from build123d import *

# Parameters (mm, degrees)
BOSS_EXTRUDE1_DEPTH      = 1.25
SKETCH2_W                = 14.25
SKETCH2_H                = 15
BOSS_EXTRUDE2_DEPTH      = 4.6
FILLET1_R                = 3
SKETCH5_W                = 20
SKETCH5_H                = 82.2
BASE_PLATE_DEPTH         = 6
SLOT_CUT_DEPTH           = 82.2
REAR_TAB_DEPTH           = 4.4
REAR_TAB_DEPTH_BACK      = 0.4
SKETCH8_W                = 15.25
SKETCH8_H                = 3
SKETCH22_W               = 15.25
SKETCH22_H               = 3
FRONT_SUPPORT_RAIL_DEPTH = 2.1
SKETCH23_W               = 0.8
SKETCH23_H               = 25
BEND_SLOT_DEPTH          = 91.682082023
SKETCH20_W               = 7.75
SKETCH20_H               = 6
SKETCH20_W_2             = 4.75
BOSS_EXTRUDE3_DEPTH      = 0.45
FILLET6_R                = 2.5
CUT_EXTRUDE4_DEPTH       = 92.879282213
CUT_EXTRUDE5_DEPTH       = 5.2
FILLET5_R                = 1
FILLET7_R                = 0.4
BOSS_EXTRUDE4_DEPTH      = 2
CHAMFER1_SIZE            = 2
FILLET8_R                = 2


# Some blends are built 0.0001 mm under size
with BuildPart() as part:
    # Sketch1 → Boss-Extrude1 (new body)
    with BuildSketch(Plane.XY):
        Polygon((0, 0), (14, 0), (14, 17), (-2, 17), (-2, 0), align=None)
    extrude(amount=BOSS_EXTRUDE1_DEPTH)

    # Sketch2 → Boss-Extrude2 (add)
    with BuildSketch(Plane.XY):
        with Locations((5.125, 7.5)):
            Rectangle(SKETCH2_W, SKETCH2_H)
    extrude(amount=-BOSS_EXTRUDE2_DEPTH)

    # Fillet1
    fillet1_edges = [part.edges().sort_by_distance(p)[0] for p in [
        (12.25, 15, -2.3),
        (14, 17, 0.625),
    ]]
    fillet(fillet1_edges, radius=FILLET1_R)

    # Mirror1: part across plane


with BuildPart() as body_2:
    # Sketch5 → Base Plate (new body)
    with BuildSketch(Plane(origin=(0, 0, 0), x_dir=(1, 0, 0), z_dir=(0, 1, 0))):
        with Locations((10, 45.7)):
            Rectangle(SKETCH5_W, SKETCH5_H)
    extrude(amount=BASE_PLATE_DEPTH)

    # Sketch18 → Slot Cut (cut)
    with BuildSketch(Plane(origin=(0, 0, -86.8), x_dir=(-1, 0, 0), z_dir=(0, 0, -1))):
        Polygon((0, 0.4), (-15.25, 0.4), (-15.25, 2.5), (-17.25, 2.5), (-17.25, 4.5), (-15.25, 6), (0, 6), align=None)
    extrude(amount=-SLOT_CUT_DEPTH, mode=Mode.SUBTRACT)

    # Sketch8 → Rear Tab (add, two sides: drawn at the far end of the back side and taken through both)
    with BuildSketch(Plane(origin=(0, 0.4, 0), x_dir=(1, 0, 0), z_dir=(0, 1, 0)).offset(-REAR_TAB_DEPTH_BACK)):
        with Locations((7.625, 85.3)):
            Rectangle(SKETCH8_W, SKETCH8_H)
    extrude(amount=REAR_TAB_DEPTH + REAR_TAB_DEPTH_BACK)

    # Sketch22 → Front Support Rail (add)
    with BuildSketch(Plane(origin=(0, 0.4, 0), x_dir=(1, 0, 0), z_dir=(0, 1, 0))):
        with Locations((7.625, 6.1)):
            Rectangle(SKETCH22_W, SKETCH22_H)
    extrude(amount=FRONT_SUPPORT_RAIL_DEPTH)

    # Sketch23 → Bend Slot (cut, through all)
    with BuildSketch(Plane(origin=(0, 0, 0), x_dir=(1, 0, 0), z_dir=(0, 1, 0))):
        with Locations((14.85, 74.3)):
            Rectangle(SKETCH23_W, SKETCH23_H)
    extrude(amount=BEND_SLOT_DEPTH, mode=Mode.SUBTRACT)

    # Mirror2: body 2 across plane


with BuildPart() as part_1:
    add(part.part)
    add(part.part.mirror(Plane(origin=(-2, 0, 1.25), x_dir=(0, 0, 1), z_dir=(1, 0, 0))))



with BuildPart() as body_2_1:
    add(body_2.part)
    add(body_2.part.mirror(Plane(origin=(0, 6, -4.6), x_dir=(0, 0, 1), z_dir=(1, 0, 0))))


with BuildPart() as part_2:
    add(part_1.part)

    add(body_2_1.part)  # Boss-Extrude3 merges body 2
    # Sketch20 → Boss-Extrude3 (add)
    with BuildSketch(Plane.XY.offset(-4.6)):
        with Locations((16.125, 3)):
            Rectangle(SKETCH20_W, SKETCH20_H)
        with Locations((-17.625, 3)):
            Rectangle(SKETCH20_W_2, SKETCH20_H)
    extrude(amount=BOSS_EXTRUDE3_DEPTH)

    # Fillet6
    fillet6_edges = [part_2.edges().sort_by_distance(p)[0] for p in [
        (-20, 3, -4.15),
        (20, 3, -4.15),
        (20, 3, -86.8),
        (0, 4.8, -86.8),
        (-20, 3, -86.8),
    ]]
    fillet(fillet6_edges, radius=FILLET6_R)

    # Sketch15 → Cut-Extrude4 (cut, through all)
    with BuildSketch(Plane.XY.offset(1.25)):
        with BuildLine():
            Line((7.5, 5), (-11.5, 5))
            ThreePointArc((-11.5, 5), (-14.5, 8), (-11.5, 11))
            Line((-11.5, 11), (7.5, 11))
            ThreePointArc((7.5, 11), (10.5, 8), (7.5, 5))
        make_face()
    extrude(amount=-CUT_EXTRUDE4_DEPTH, mode=Mode.SUBTRACT)

    # Sketch16 → Cut-Extrude5 (cut)
    with BuildSketch(Plane.XY.offset(1.25)):
        with BuildLine():
            Line((-15.6, 0), (11.6, 0))
            Line((11.6, 0), (11.6, 12))
            ThreePointArc((11.6, 12), (10.911700936, 13.661700936), (9.25, 14.35))
            Line((9.25, 14.35), (-13.25, 14.35))
            ThreePointArc((-13.25, 14.35), (-14.911700936, 13.661700936), (-15.6, 12))
            Line((-15.6, 12), (-15.6, 0))
        make_face()
    extrude(amount=-CUT_EXTRUDE5_DEPTH, mode=Mode.SUBTRACT)

    # Fillet5
    # the kernel refuses this fillet: 1 mm, written as the material it adds along each edge
    with BuildSketch(Plane(origin=(9.25, 14.35, -3.95), x_dir=(0, -1, 0), z_dir=(-1, 0, 0))) as fillet5_piece_1:
        with BuildLine():
            CenterArc((FILLET5_R, FILLET5_R), FILLET5_R, 180, 90)
            Line((0, FILLET5_R), (0, 0))
            Line((0, 0), (FILLET5_R, 0))
        make_face()
    extrude(amount=22.5)
    with BuildSketch(Plane(origin=(-13.25, 12, -3.95), x_dir=(0, 1, 0), z_dir=(1, 0, 0))) as fillet5_piece_2:
        with BuildLine():
            CenterArc((2.35 - FILLET5_R, FILLET5_R), FILLET5_R, 270, 90)
            Line((2.35, FILLET5_R), (2.35, 0))
            Line((2.35, 0), (2.35 - FILLET5_R, 0))
        make_face()
    revolve(axis=Axis((-13.25, 12, -3.95), (0, 0, 1)), revolution_arc=90)
    with BuildSketch(Plane(origin=(-15.6, 12, -3.95), x_dir=(1, 0, 0), z_dir=(0, -1, 0))) as fillet5_piece_3:
        with BuildLine():
            CenterArc((FILLET5_R, FILLET5_R), FILLET5_R, 180, 90)
            Line((0, FILLET5_R), (0, 0))
            Line((0, 0), (FILLET5_R, 0))
        make_face()
    extrude(amount=12)
    with BuildSketch(Plane(origin=(11.6, 0, -3.95), x_dir=(0, 0, 1), z_dir=(0, 1, 0))) as fillet5_piece_4:
        with BuildLine():
            CenterArc((FILLET5_R, -FILLET5_R), FILLET5_R, 90, 90)
            Line((0, -FILLET5_R), (0, 0))
            Line((0, 0), (FILLET5_R, 0))
        make_face()
    extrude(amount=12)
    with BuildSketch(Plane(origin=(9.25, 12, -3.95), x_dir=(1, 0, 0), z_dir=(0, -1, 0))) as fillet5_piece_5:
        with BuildLine():
            CenterArc((2.35 - FILLET5_R, FILLET5_R), FILLET5_R, 270, 90)
            Line((2.35, FILLET5_R), (2.35, 0))
            Line((2.35, 0), (2.35 - FILLET5_R, 0))
        make_face()
    revolve(axis=Axis((9.25, 12, -3.95), (0, 0, 1)), revolution_arc=90)
    with BuildSketch(Plane(origin=(15.25, 0.4, -7.6), x_dir=(0, 0, -1), z_dir=(0, 1, 0))) as fillet5_piece_6:
        with BuildLine():
            CenterArc((FILLET5_R, FILLET5_R), FILLET5_R, 180, 90)
            Line((0, FILLET5_R), (0, 0))
            Line((0, 0), (FILLET5_R, 0))
        make_face()
    extrude(amount=2.1)
    with BuildSketch(Plane(origin=(-15.25, 0.4, -7.6), x_dir=(0, 0, -1), z_dir=(0, 1, 0))) as fillet5_piece_7:
        with BuildLine():
            CenterArc((FILLET5_R, -FILLET5_R), FILLET5_R, 90, 90)
            Line((0, -FILLET5_R), (0, 0))
            Line((0, 0), (FILLET5_R, 0))
        make_face()
    extrude(amount=2.1)
    # the kernel refuses this fillet: 1 mm, written as the material it takes off along each edge
    with BuildSketch(Plane(origin=(17.25, 2.5, -86.8), x_dir=(0.9759656656854916, -1.7336632852602407e-15, 0.21792434330077798), z_dir=(0, 1, 0))) as fillet5_2_piece_1_section:
        with BuildLine():
            CenterArc((1.237684498, -0.954173231), FILLET5_R, 72.587148881, 120)
            Line((0.261718832, -1.172097575), (0.164122266, -1.193890009))
            Line((0.164122266, -1.193890009), (-0.097596567, -0.021792434))
            Line((-0.097596567, -0.021792434), (-0.021792434, 0.097596567))
            ThreePointArc((-0.021792434, 0.097596567), (0.222198982, 0.152077652), (1.566864795, 0.095417323))
            Line((1.566864795, 0.095417323), (1.536939313, 0))
        make_face()
    fillet5_2_piece_1 = extrude(amount=5.842348283, mode=Mode.PRIVATE)
    fillet5_2_piece_1 = split(fillet5_2_piece_1, bisect_by=Plane(origin=(18.04936, 3.90048, -86.46679556), z_dir=(-0.5999999999999985, -0.8000000000000012, 0)), keep=Keep.TOP, mode=Mode.PRIVATE)
    add(fillet5_2_piece_1, mode=Mode.SUBTRACT)
    with BuildSketch(Plane(origin=(-17.25, 2.5, -86.8), x_dir=(-0.9759656656854916, -1.7336632852602407e-15, 0.21792434330077798), z_dir=(0, 1, 0))) as fillet5_2_piece_2_section:
        with BuildLine():
            CenterArc((1.237684498, 0.954173231), FILLET5_R, 167.412851119, 120)
            Line((0.261718832, 1.172097575), (0.164122266, 1.193890009))
            Line((0.164122266, 1.193890009), (-0.097596567, 0.021792434))
            Line((-0.097596567, 0.021792434), (-0.021792434, -0.097596567))
            ThreePointArc((-0.021792434, -0.097596567), (0.222198982, -0.152077652), (1.566864795, -0.095417323))
            Line((1.566864795, -0.095417323), (1.536939313, 0))
        make_face()
    fillet5_2_piece_2 = extrude(amount=5.842348283, mode=Mode.PRIVATE)
    fillet5_2_piece_2 = split(fillet5_2_piece_2, bisect_by=Plane(origin=(-18.04936, 3.90048, -86.46679556), z_dir=(0.5999999999999985, -0.8000000000000012, 0)), keep=Keep.TOP, mode=Mode.PRIVATE)
    add(fillet5_2_piece_2, mode=Mode.SUBTRACT)

    # Fillet7
    fillet7_edges = [part_2.edges().sort_by_distance(p)[0] for p in [
        (-14.45, 0.2, -61.8),
        (-15.25, 0.2, -61.8),
        (14.45, 0.2, -61.8),
        (15.25, 0.2, -61.8),
    ]]
    fillet(fillet7_edges, radius=FILLET7_R - 0.0001)  # a hair under: the kernel refuses the full size

    # Sketch24 → Boss-Extrude4 (add)
    with BuildSketch(Plane(origin=(0, 0, -4.6), x_dir=(-1, 0, 0), z_dir=(0, 0, -1))):
        Polygon((-9.25, 15), (-9.25, 17), (13.25, 17), (13.25, 15), (13.25, 13), (-9.25, 13), align=None)
    extrude(amount=BOSS_EXTRUDE4_DEPTH)

    # Chamfer1
    chamfer1_edges = [part_2.edges().sort_by_distance(p)[0] for p in [
        (-2, 13, -6.6),
    ]]
    chamfer(chamfer1_edges, length=CHAMFER1_SIZE - 0.0001)  # a hair under: the kernel refuses the full size

    # Fillet8
    fillet8_edges = [part_2.edges().sort_by_distance(p)[0] for p in [
        (-13.25, 17, -5.6),
        (9.25, 17, -5.6),
    ]]
    fillet(fillet8_edges, radius=FILLET8_R)


solid = part_2.part
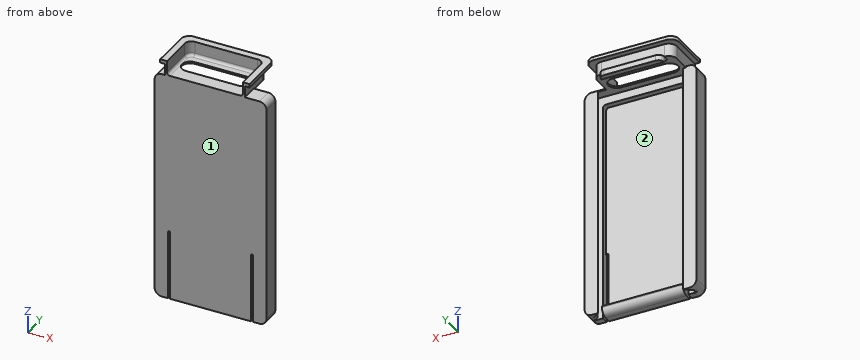
Read the model definition and answer for the solid it produces. Units are mm, in the model's axes. Face numbers are marked on the shaded views. Round coordinates to 2 decimals unless told otherwise and drop trailing zeros. Order: outer loops, then holes, each group sorted by start corner. A loop starts at its lowest first (then second) coordinate and runs counter-clockwise, first axis right, second up.
1) The part is cut by section B-B on y = 8. Write down the section's boundary in (x, z), plus the area to 3 significant figures.
2) Flat-ended cylindrical pins translate along their axes: pin 1 (1 mm diameter, centred on y = 7.5, z = 1, fed in from +X); pin 2 (1.6 mm diameter, centred on y = 14, z = -6, fed in from -X); pin 3 (1.5 mm diameter, centred on x = -8.5, y = 4.5, fed in from -Z). Find the tip coordinate at first contact, or state that the pin passes through.
3) The part is cut by section C-C on z = -65.5. Write down the section's boundary in (x, y).
4) The part is cut by section D-D on z = -13. Write down the section's boundary in (x, y).
5) Straight lines are drawn through the part: L1, parallel to Z at x = -8.5, y = 2; L2, parallel to Z at x = 9, y = 15.5; L3, parallel to X at y = 1, z = -82. For each, find the intervals that lie inside material, in ascending order.
6) The mould has two halves that part along X. Classify the marked faces 1 and 2: released by +X, released by -X, zero draft, split by the parting line, or undercut.
Resolved:
1. outline: (-18, 0) - (-16.25, 0) - (-16.25, -4.6) - (-14.5, -4.6) - (-14.5, -3.95) - (-14.6, -3.95) arc R1 cw to (-15.6, -2.95) - (-15.6, 1.25) - (-18, 1.25) - close; (10.5, -4.6) - (12.25, -4.6) - (12.25, 0) - (14, 0) - (14, 1.25) - (11.6, 1.25) - (11.6, -2.95) arc R1 cw to (10.6, -3.95) - (10.5, -3.95) - close
1. area: 13.8 mm2
2. pin 1: stops at x = 14
2. pin 2: stops at x = -13.25
2. pin 3: stops at z = -86.34
3. outline: (-20, 0) - (-15.25, 0) - (-15.25, 2.5) - (-17.25, 2.5) - (-17.25, 4.5) - (-15.25, 6) - (-20, 6) - close; (-14.45, 0) - (14.45, 0) - (14.45, 0.4) - (-14.45, 0.4) - close; (15.25, 0) - (20, 0) - (20, 6) - (15.25, 6) - (17.25, 4.5) - (17.25, 2.5) - (15.25, 2.5) - close
4. outline: (-20, 0) - (20, 0) - (20, 6) - (15.25, 6) - (17.25, 4.5) - (17.25, 2.5) - (15.25, 2.5) - (15.25, 0.4) - (-15.25, 0.4) - (-15.25, 2.5) - (-17.25, 2.5) - (-17.25, 4.5) - (-15.25, 6) - (-20, 6) - close
5. L1: z = -86.8 to -83.8, -7.6 to -3.95
5. L2: z = -6.6 to -4.6, 0 to 1.25
5. L3: x = -20 to -15.25, 15.25 to 20
6. face 1: zero draft
6. face 2: undercut
